Check sheet for the modelled part. Datum: model origin and axes. Units: mm. A direction names the side the tool comes from. Round coordinates to 2 decimals unless told otherwise and drop trailing zeros. Order: outer loops, then holes, each group sorted by start corner. A loop starts at its lowest first (then second) coordinate and runs counter-clockwise, first axis right, second up. Notation, with made-up numbers: (-20, -7.75) -> (38, -7.75) arc R18 cw to (38, 24.25) -> close; hole circle Ø3 at (70, 67.25). An arc over 180 degrees is marked (long way). Answer in a Markdown table with one row per item.
from build123d import *

# Parameters (mm, degrees)
SKETCH2_R               = 25
BOSS_EXTRUDE1_DEPTH     = 20
SKETCH3_R               = 25
BOSS_EXTRUDE2_DEPTH     = 100
CUT_EXTRUDE1_DEPTH      = 188.082869339
CUT_EXTRUDE1_DEPTH_BACK = 188.082869339
SKETCH4_W               = 40
SKETCH4_H               = 100


with BuildPart() as part:
    # Sketch2 → Boss-Extrude1 (new, symmetric)
    with BuildSketch(Plane(origin=(0, 0, 0), x_dir=(0, 0, -1), z_dir=(1, 0, 0))):
        with BuildLine():
            Line((-50, 0), (50, 0))
            Line((50, 0), (50, -100))
            ThreePointArc((50, -100), (0, -150), (-50, -100))
            Line((-50, -100), (-50, 0))
        make_face()
        with Locations((0, -100)):
            Circle(SKETCH2_R, mode=Mode.SUBTRACT)
    extrude(amount=BOSS_EXTRUDE1_DEPTH, both=True)

    # Sketch3 → Boss-Extrude2 (add)
    with BuildSketch(Plane(origin=(0, 0, -50), x_dir=(-1, 0, 0), z_dir=(0, 0, -1))):
        with BuildLine():
            Line((-50, 0), (50, 0))
            Line((50, 0), (50, 100))
            ThreePointArc((50, 100), (0, 150), (-50, 100))
            Line((-50, 100), (-50, 0))
        make_face()
        with Locations(Location((0, 100, 0), (0, 0, 90))):
            Circle(SKETCH3_R, mode=Mode.SUBTRACT)
    extrude(amount=-BOSS_EXTRUDE2_DEPTH)

    # Sketch4 → Cut-Extrude1 (cut, two sides: drawn at the far end of the back side and taken through both)
    with BuildSketch(Plane(origin=(50, 0, 0), x_dir=(0, 0, -1), z_dir=(1, 0, 0)).offset(-CUT_EXTRUDE1_DEPTH_BACK)):
        with Locations((1.706579079, 100)):
            Rectangle(SKETCH4_W, SKETCH4_H)
    extrude(amount=CUT_EXTRUDE1_DEPTH + CUT_EXTRUDE1_DEPTH_BACK, mode=Mode.SUBTRACT)


solid = part.part
Item 1: Depth check by flat-ended pin: P1, Ø5, axis at x = 33.5, z = 22.5, coming from the +Y side; P2, Ø9, axis at x = -28.5, z = 16.5, coming from the -Y side; P3, Ø5, axis at x = -1, z = -3.5, coming from the -Y side. Enter the tip coordinate at first touch or a pass-through.
Result sheet:
| item | result |
|---|---|
| P1 | stops at y = 139.23 |
| P2 | stops at y = 0 |
| P3 | stops at y = -149.99 |
Item 2: Scan lines: line 1 (X direction, y = 100, z = -43); line 2 (Z direction, x = 46.5, y = 59.5); line 3 (Y direction, x = 21.5, z = 5). Record each from-to range of solid material in increasing order. Write a range as [from, to].
Result sheet:
| item | result |
|---|---|
| line 1 | x = [-50, -25], [25, 50] |
| line 2 | z = [-50, -21.71], [18.29, 50] |
| line 3 | y = [0, 50] |
Item 3: Cross-section at C-C (y = 71). Record the boundary of the cut face in (x, z), and give its area (3 significant figures).
Result sheet:
| item | result |
|---|---|
| outline | (-50, -50) -> (50, -50) -> (50, -21.71) -> (-50, -21.71) -> close; (-50, 18.29) -> (50, 18.29) -> (50, 50) -> (-50, 50) -> close |
| area | 6,000 mm^2 |
Item 4: Set-up check for faces 4 (the flat face through (20, -57, -1)), 5 (the cylindrical face through (1.099, 75.024, 33.925)), 6 (the flat face through (-35, 0, -1)), 7 (the flat face through (-12, 77, 18.293)): record each of +Z, -Z, +X, -X, +Y, -Y from which the full face is reachable in a straight line by a thin tool's end or side.
Result sheet:
| item | result |
|---|---|
| face 4 | +Z, -Z, +X, -Y |
| face 5 | +Z, -Z |
| face 6 | +Z, -Z, -X, -Y |
| face 7 | +X, -X, +Y |
Item 5: Mould release check, pull along Z, two halves, no side actions. Record for faces 1 (the cylindrical face through (-0.28, -124.406, 5.42)), 2 (the cylindrical face through (0.28, -149.988, -1.099)), 3 (the flat face through (50, 40, -1)): pulls with the +Z half, pulls with the -Z half, needs draft (parallel to the pull), parting line crosses it, or undercut.
Result sheet:
| item | result |
|---|---|
| face 1 | undercut |
| face 2 | parting line crosses it |
| face 3 | needs draft |
Item 6: Cross-section at B-B (z = 0). Record the boundary of the cut face in (x, y).
Result sheet:
| item | result |
|---|---|
| outline | (-50, 0) -> (-20, 0) -> (-20, -75) -> (20, -75) -> (20, 0) -> (50, 0) -> (50, 50) -> (-50, 50) -> close; (-20, -150) -> (20, -150) -> (20, -125) -> (-20, -125) -> close |
Item 7: Cross-section at A-A (x = 0). Record the boundary of the cut face in (y, z), and give its area (3 significant figures).
Result sheet:
| item | result |
|---|---|
| outline | (-100, -50) -> (75, -50) -> (75, -21.71) -> (50, -21.71) -> (50, 18.29) -> (75, 18.29) -> (75, 50) -> (-100, 50) arc R50 ccw to start; (125, -50) -> (150, -50) -> (150, -21.71) -> (125, -21.71) -> close; (125, 18.29) -> (150, 18.29) -> (150, 50) -> (125, 50) -> close; hole circle Ø50 at (-100, 0) |
| area | 20,000 mm^2 |
Item 8: Cross-section at D-D (z = 30.5). Record the boundary of the cut face in (x, y).
Result sheet:
| item | result |
|---|---|
| outline | (-50, 0) -> (-20, 0) -> (-20, -139.62) -> (20, -139.62) -> (20, 0) -> (50, 0) -> (50, 100) arc R50 ccw to (-50, 100) -> close; hole circle Ø50 at (0, 100) |
